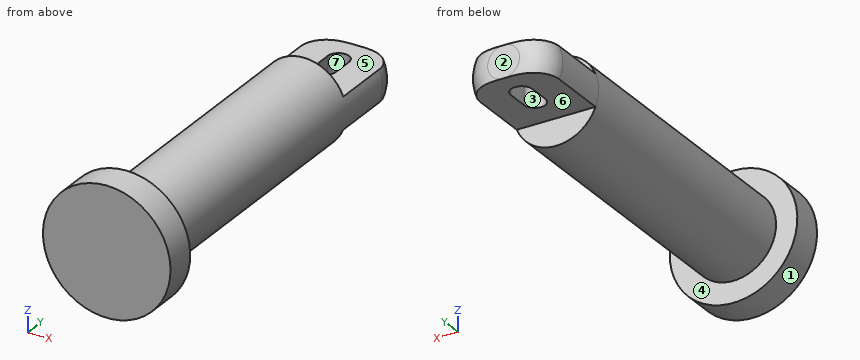
from build123d import *

# Parameters (mm, degrees)
SKETCH1_R           = 3
BOSS_EXTRUDE1_DEPTH = 1.5
SKETCH2_R           = 2
BOSS_EXTRUDE2_DEPTH = 13.5
BOSS_EXTRUDE3_DEPTH = 4
CUT_EXTRUDE1_DEPTH  = 3
FILLET5_R           = 1.25


with BuildPart() as part:
    # Sketch1 → Boss-Extrude1 (new body)
    with BuildSketch(Plane(origin=(0, 0, 0), x_dir=(1, 0, 0), z_dir=(0, 1, 0))):
        with Locations(Location((0, 0, 0), (0, 0, 270))):
            Circle(SKETCH1_R)
    extrude(amount=BOSS_EXTRUDE1_DEPTH)

    # Sketch2 → Boss-Extrude2 (add)
    with BuildSketch(Plane(origin=(0, 1.5, 0), x_dir=(1, 0, 0), z_dir=(0, 1, 0))):
        with Locations(Location((0, 0, 0), (0, 0, 270))):
            Circle(SKETCH2_R)
    extrude(amount=BOSS_EXTRUDE2_DEPTH)

    # Sketch6 → Boss-Extrude3 (add)
    with BuildSketch(Plane(origin=(0, 15, 0), x_dir=(1, 0, 0), z_dir=(0, 1, 0))):
        with BuildLine():
            Line((1.854049622, 0.75), (-1.854049622, 0.75))
            ThreePointArc((-1.854049622, 0.75), (-2, 0), (-1.854049622, -0.75))
            Line((-1.854049622, -0.75), (1.854049622, -0.75))
            ThreePointArc((1.854049622, -0.75), (2, 0), (1.854049622, 0.75))
        make_face()
    extrude(amount=BOSS_EXTRUDE3_DEPTH)

    # Sketch7 → Cut-Extrude1 (cut)
    with BuildSketch(Plane.XY.offset(0.75)):
        with BuildLine():
            Line((-0.5, 16.62671351), (-0.5, 17.62671351))
            ThreePointArc((-0.5, 17.62671351), (0, 18.12671351), (0.5, 17.62671351))
            Line((0.5, 17.62671351), (0.5, 16.62671351))
            ThreePointArc((0.5, 16.62671351), (0, 16.12671351), (-0.5, 16.62671351))
        make_face()
    extrude(amount=-CUT_EXTRUDE1_DEPTH, mode=Mode.SUBTRACT)

    # Fillet5
    fillet5_edges = [part.edges().sort_by_distance(p)[0] for p in [
        (-2, 19, 0),
        (2, 19, 0),
    ]]
    fillet(fillet5_edges, radius=FILLET5_R - 0.0001)  # a hair under: the kernel refuses the full size


solid = part.part
Could you check a few things on this model? Use its own coordinates, in mm. Face numbers are marked on the shaded views. A direction names the side the tool comes from. Coordinates: 2 decimals unless noted, no trailing zeros. Order: outer loops, then holes, each group sorted by start corner. A loop starts at its lowest first (then second) coordinate and runs counter-clockwise, first axis right, second up.
Q1. Suppose I cut it at B-B on y = 12.5. Please give me the cut outline in (x, z), and give its area (3 significant figures).
Q2. Which directions (+Z, -Z, +X, -X, +Y, -Y) give clear straight access to the entire face, cutting with the end or side of a thin tool? Please do the marked faces 4, 5, 6 and 7.
Q3. Thinking about a two-plate mould opening in Y: for the marked faces 1, 2 and 3, which applies, released by +Y, released by -Y, zero draft, split by the parting line, or undercut?
Q4. Please list where these lines run through material, in increasing order: L1, parallel to Y at x = 0, z = -0.1; L2, parallel to Y at x = 0.5, z = -2.05; L3, parallel to Z at x = -0.7, y = 17.75.
Q5. Suppose I cut it at D-D on z = 2.4. Please give me the cut outline in (x, y), and give its area (3 significant figures).
Q6. Will these pins go through, and if not, where does the flat tip stop? pin 1 (0.6 mm diameter, centred on x = 0.5, z = 1.5, fed in from +Y); pin 2 (3 mm diameter, centred on y = 4.5, z = 1, fed in from +X); pin 3 (3 mm diameter, centred on y = 8.5, z = -1, fed in from -X).
Q7. Suppose I cut it at A-A on z = -1.75. Please give me the cut outline in (x, y).
Q8. Suppose I cut it at C-C on z = 1.25. Please give me the cut outline in (x, y), and give its area (3 significant figures).
Answer:
1. outline: circle Ø4 at (0, 0)
1. area: 12.6 mm2
2. face 4: +Y
2. face 5: +Z, +X, -X, +Y
2. face 6: -Z, +X, -X, +Y
2. face 7: +Z, -Z
3. face 1: zero draft
3. face 2: released by +Y
3. face 3: undercut
4. L1: y = 0 to 16.13, 18.13 to 19
4. L2: y = 0 to 1.5
4. L3: z = -0.75 to 0.75
5. outline: (-1.8, 0) - (1.8, 0) - (1.8, 1.5) - (-1.8, 1.5) - close
5. area: 5.40 mm2
6. pin 1: stops at y = 15
6. pin 2: stops at x = 2
6. pin 3: stops at x = -2
7. outline: (-2.44, 0) - (2.44, 0) - (2.44, 1.5) - (0.97, 1.5) - (0.97, 15) - (-0.97, 15) - (-0.97, 1.5) - (-2.44, 1.5) - close
8. outline: (-2.73, 0) - (2.73, 0) - (2.73, 1.5) - (1.56, 1.5) - (1.56, 15) - (-1.56, 15) - (-1.56, 1.5) - (-2.73, 1.5) - close
8. area: 50.3 mm2
